Could you check a few things on this model? Use its own coordinates, in mm. A direction names the side the tool comes from. Give positions to 0.01 mm unless a question says otherwise; leave off trailing zeros. Order: outer loops, then holes, each group sorted by start corner. A loop starts at its lowest first (then second) coordinate and runs counter-clockwise, first axis right, second up. Notation, with made-up numbers: M -28.5,-32 L -20.5,-32 A31 cw -20.5,-1 Z; hole C -0.75,33.25 d1. An arc over 180 degrees is marked long. Use a Markdown table: item, result. Add a question column.
Item 1: For faces 3 (the face through (-0.1, 12.8, 7)), 4 (the face through (-0.1, 12.8, -8)), 5 (the face through (0, 10, 0)), which set-ups out of +Z, -Z, +X, -X, +Y, -Y let a thin tool reach every point of the face, with its end or its side?
Item 2: If I drill on L1, parallel to Y at x = 0, z = 0; L2, parallel to Y at x = -5.5, z = 4.5; L3, parallel to Z at x = -8, y = 5.5, over which ranges is the centre line in solid material (lowest first)? Write a range as from..to.
Item 3: If we mould it in two halves opening along X, with no side actions, what happens to faces 1 (the face through (-8, 24, 0)), 2 (the face through (-0.217, 13.144, -0.395))? For each: released by +X, released by -X, zero draft, split by the parting line, or undercut.
Item 4: Suppose I cut it at C-C on x = 3.5. Write out the boundary of the cut face in (y, z), plus the area to 3 significant figures.
Item 5: I'm going to push flat-ended pins straight in: pin 1 Ø1.5 at (y, z) = (15.5, 5.5) entering from +X; pin 2 Ø1.5 at (x, y) = (0, 19) entering from -Z; pin 3 Ø10 at (x, y) = (1, 11) entering from -Z; pin 4 Ø4 at (y, z) = (9, -6.5) entering from -X. Where does each tip first touch, or does it pass through?
Item 6: Suppose I cut it at B-B on x = 0. Write out the boundary of the cut face in (y, z).
Item 7: Suppose I cut it at A-A on y = 7. Write out the boundary of the cut face in (x, z), plus the area to 3 significant figures.
Item 8: Suppose I cut it at D-D on y = 10.5. Write out the boundary of the cut face in (x, z), plus the area to 3 significant figures.
from build123d import *

# Parameters (mm, degrees)
SKETCH1_R           = 10
BOSS_EXTRUDE1_DEPTH = 4
BOSS_EXTRUDE2_DEPTH = 20
SKETCH6_W           = 12
SKETCH6_H           = 15
BOSS_EXTRUDE4_DEPTH = 3
SKETCH10_W          = 12
SKETCH10_H          = 15
BOSS_EXTRUDE5_DEPTH = 4
FILLET1_R           = 1
CUT_EXTRUDE3_REACH  = 33.064
SKETCH7_R           = 1


with BuildPart() as part:
    # Sketch1 → Boss-Extrude1 (new body)
    with BuildSketch(Plane(origin=(0, 0, 0), x_dir=(1, 0, 0), z_dir=(0, 1, 0))):
        with Locations(Location((0, 0, 0), (0, 0, 270))):
            Circle(SKETCH1_R)
    extrude(amount=BOSS_EXTRUDE1_DEPTH)

    # Sketch2 → Boss-Extrude2 (add)
    with BuildSketch(Plane(origin=(0, 4, 0), x_dir=(1, 0, 0), z_dir=(0, 1, 0))):
        with BuildLine():
            Line((-6, 7.7), (-6, -7.7))
            ThreePointArc((-6, -7.7), (-6.145446182, -7.798029265), (-6.315135994, -7.753648005))
            ThreePointArc((-6.315135994, -7.753648005), (-10, 0), (-6.315135994, 7.753648005))
            ThreePointArc((-6.315135994, 7.753648005), (-6.145446182, 7.798029265), (-6, 7.7))
        make_face()
        with BuildLine():
            Line((6, 7.6), (6, -7.7))
            ThreePointArc((6, -7.7), (6.145446182, -7.798029265), (6.315135994, -7.753648005))
            ThreePointArc((6.315135994, -7.753648005), (9.999874962, 0.050007502), (6.237272998, 7.816420251))
            ThreePointArc((6.237272998, 7.816420251), (6.069665116, 7.76190005), (6, 7.6))
        make_face()
    extrude(amount=BOSS_EXTRUDE2_DEPTH)

    # Sketch6 → Boss-Extrude4 (add)
    with BuildSketch(Plane(origin=(0, 14, 0), x_dir=(1, 0, 0), z_dir=(0, 1, 0))):
        with Locations((0, 0.5)):
            Rectangle(SKETCH6_W, SKETCH6_H)
    extrude(amount=BOSS_EXTRUDE4_DEPTH)

    # Sketch10 → Boss-Extrude5 (add)
    with BuildSketch(Plane.XZ.offset(-14)):
        with Locations((0, -0.5)):
            Rectangle(SKETCH10_W, SKETCH10_H)
    extrude(amount=BOSS_EXTRUDE5_DEPTH)

    # Fillet1
    # the kernel refuses this fillet: 1 mm, written as the material it takes off along each edge
    with BuildSketch(Plane(origin=(6, 14, -8), x_dir=(0, 0, 1), z_dir=(0, -1, 0))) as fillet1_piece_1_section:
        with BuildLine():
            CenterArc((1, 0.793964744), FILLET1_R, 180, 52.557582208)
            Line((0, 0.793964744), (-0.02, 0.793964744))
            Line((-0.02, 0.793964744), (-0.02, 0))
            Line((-0.02, 0), (0, -0.02))
            ThreePointArc((0, -0.02), (0.196018099, -0.02), (0.379876922, -0.015879295))
            Line((0.379876922, -0.015879295), (0.392036198, 0))
        make_face()
    fillet1_piece_1 = extrude(amount=5.984911861, mode=Mode.PRIVATE)
    fillet1_piece_1 = fillet1_piece_1 - Plane(origin=(6.213704622, 11.00754407, -7.603981901), x_dir=(0.11026568498271415, 0, -0.993902147454815), z_dir=(0, -1, 0)) * Cylinder(0.213741715, 16, mode=Mode.PRIVATE)
    add(fillet1_piece_1, mode=Mode.SUBTRACT)
    with BuildSketch(Plane(origin=(-6, 14, -8), x_dir=(0, 0, 1), z_dir=(0, -1, 0))) as fillet1_piece_2_section:
        with BuildLine():
            CenterArc((1, -0.714142843), FILLET1_R, 134.427004001, 45.572995999)
            Line((0, -0.714142843), (-0.02, -0.714142843))
            Line((-0.02, -0.714142843), (-0.02, 0))
            Line((-0.02, 0), (0, 0.02))
            ThreePointArc((0, 0.02), (0.15, 0.02), (0.286, 0.014282857))
            Line((0.286, 0.014282857), (0.3, 0))
        make_face()
    fillet1_piece_2 = extrude(amount=5.785357107, mode=Mode.PRIVATE)
    fillet1_piece_2 = fillet1_piece_2 - Plane(origin=(-6.181186106, 11.107321446, -7.588087879), x_dir=(-0.628985521858462, 0, -0.7774170137657384), z_dir=(0, -1, 0)) * Cylinder(0.212961798, 15, mode=Mode.PRIVATE)
    add(fillet1_piece_2, mode=Mode.SUBTRACT)
    with BuildSketch(Plane(origin=(-6, 14, -8), x_dir=(0, 0, 1), z_dir=(0, 1, 0))) as fillet1_piece_3_section:
        with BuildLine():
            CenterArc((1, 0.714142843), FILLET1_R, 180, 45.572995999)
            Line((0, 0.714142843), (-0.02, 0.714142843))
            Line((-0.02, 0.714142843), (-0.02, 0))
            Line((-0.02, 0), (0, -0.02))
            ThreePointArc((0, -0.02), (0.15, -0.02), (0.286, -0.014282857))
            Line((0.286, -0.014282857), (0.3, 0))
        make_face()
    fillet1_piece_3 = extrude(amount=4.785357107, mode=Mode.PRIVATE)
    fillet1_piece_3 = fillet1_piece_3 - Plane(origin=(-6.181186106, 16.392678554, -7.588087879), x_dir=(-0.628985521858462, 0, -0.7774170137657384), z_dir=(0, -1, 0)) * Cylinder(0.212961798, 13, mode=Mode.PRIVATE)
    add(fillet1_piece_3, mode=Mode.SUBTRACT)
    with BuildSketch(Plane(origin=(6, 14, -8), x_dir=(0, 0, 1), z_dir=(0, 1, 0))) as fillet1_piece_4_section:
        with BuildLine():
            CenterArc((1, -0.793964744), FILLET1_R, 127.442417792, 52.557582208)
            Line((0, -0.793964744), (-0.02, -0.793964744))
            Line((-0.02, -0.793964744), (-0.02, 0))
            Line((-0.02, 0), (0, 0.02))
            ThreePointArc((0, 0.02), (0.196018099, 0.02), (0.379876922, 0.015879295))
            Line((0.379876922, 0.015879295), (0.392036198, 0))
        make_face()
    fillet1_piece_4 = extrude(amount=4.984911861, mode=Mode.PRIVATE)
    fillet1_piece_4 = fillet1_piece_4 - Plane(origin=(6.213704622, 16.49245593, -7.603981901), x_dir=(0.11026568498271415, 0, -0.993902147454815), z_dir=(0, -1, 0)) * Cylinder(0.213741715, 14, mode=Mode.PRIVATE)
    add(fillet1_piece_4, mode=Mode.SUBTRACT)

    # Sketch7 → Cut-Extrude3 (cut, up to next)
    with BuildSketch(Plane.XY.offset(7), mode=Mode.PRIVATE) as cut_extrude3_sk1:
        with Locations((0, 14.12)):
            Circle(SKETCH7_R)
    cut_extrude3_tool1 = extrude(cut_extrude3_sk1.sketch, amount=-CUT_EXTRUDE3_REACH, mode=Mode.PRIVATE) & part.part
    add(cut_extrude3_tool1.solids().sort_by_distance((0, 14.12, 7))[0], mode=Mode.SUBTRACT)


solid = part.part
Findings below:
| question | item | result |
|---|---|---|
| 1 | face 3 | +Z, +Y |
| 1 | face 4 | -Z, +X, -X, +Y |
| 1 | face 5 | +Z, -Z |
| 2 | L1 | y = 0..4, 10..13.12, 15.12..17 |
| 2 | L2 | y = 0..4, 10..17 |
| 2 | L3 | z = -6..6 |
| 3 | face 1 | zero draft |
| 3 | face 2 | undercut |
| 4 | outline | M 0,-9.37 L 4,-9.37 L 4,9.37 L 0,9.37 Z; M 10,-8 L 17,-8 L 17,7 L 10,7 Z |
| 4 | area | 180 mm^2 |
| 5 | pin 1 | stops at x = 8.8 |
| 5 | pin 2 | passes through |
| 5 | pin 3 | stops at z = -8 |
| 5 | pin 4 | stops at x = -8.93 |
| 6 | outline | M 0,-10 L 4,-10 L 4,10 L 0,10 Z; M 10,-8 L 13.12,-8 L 13.12,7 L 10,7 Z; M 15.12,-8 L 17,-8 L 17,7 L 15.12,7 Z |
| 7 | outline | M -6.32,-7.75 A0.21 ccw -6,-7.7 L -6,7.7 A0.21 ccw -6.32,7.75 A10 ccw Z; M 6,-7.6 A0.21 ccw 6.24,-7.82 A10 ccw 6.32,7.75 A0.21 ccw 6,7.7 Z |
| 7 | area | 89.3 mm^2 |
| 8 | outline | M -6.32,-7.75 A0.21 ccw -6,-7.7 A1 ccw -5.29,-8 L 5.21,-8 A1 ccw 6,-7.61 A0.21 ccw 6.24,-7.82 A10 ccw 6.32,7.75 A0.21 ccw 6,7.7 L 6,7 L -6,7 L -6,7.7 A0.21 ccw -6.32,7.75 A10 ccw Z |
| 8 | area | 269 mm^2 |
